Could you check a few things on this model? Use its own coordinates, in mm. A direction names the side the tool comes from. Give positions to 0.01 mm unless a question says otherwise; leave off trailing zeros. Loops run counter-clockwise (first coordinate to the right, second up) from the corner with the lowest first, then second, coordinate; pieces in that order, holes last. Notation, with made-up numbers: (37, 27) - (73, 27) arc R15 ccw to (73, 52) - close; hole circle Ø9 at (52, 12.25). An arc over 180 degrees is marked (long way). Write each question's results on one line, items separated by ' | '. Start each with the question number.
(1) For pin 1 (0.8 mm diameter, centred on x = 3, z = 30.5, fed in from -Y), with a flat end and sliding along its axis, tell me the tip position at first contact or that it passes through.
(2) Suppose I cut it at D-D (y = 6). Count the separate pieces of the cut face and the enclosed holes in it, and give its area (3 significant figures).
(3) On a 3-axis mill with a long thin cutter (end or side, diameter ignored), from which of +Z, -Z, +X, -X, +Y, -Y can I reach the whole of each face in a straight line? I mean faces 3 (the face through (5.5, 14, 29)), 4 (the face through (3, 18, 2)), 5 (the face through (11.5, 7, 30)), 6 (the face through (3, 4.2, 30)), 7 (the face through (3, 10, 4.5)). Say none if no direction works.
(4) Suppose I cut it at B-B (x = 3). Please give me the cut outline in (y, z), and give its area (3 significant figures).
(5) Suppose I cut it at C-C (z = 13.5). Please give me the cut outline in (x, y).
(6) Suppose I cut it at A-A (y = 14.5). Please give me the cut outline in (x, z), and give its area (3 significant figures).
(7) I need wall thicknesses on line 1 (Y direction, x = 1.05, z = 2.25); line 2 (Y direction, x = 8.5, z = 2.25); line 3 (Z direction, x = 4, y = 17.5). Which ranges of each line are inside material? Lowest first, please.
(8) If we mould it in two halves opening along Z, with no side actions, what happens to faces 1 (the face through (12, 18, 2)), 2 (the face through (3, 4.2, 2))? For each: released by +Z, released by -Z, zero draft, split by the parting line, or undercut.
from build123d import *

# Parameters (mm, degrees)
SKETCH_1_W          = 15
SKETCH_1_H          = 32.4
SKETCH_1_R          = 0.8
EXTRUDE_1_DEPTH     = 2.2
SKETCH_2_W          = 15
SKETCH_2_H          = 32.4
SKETCH_2_W_2        = 12.4
SKETCH_2_H_2        = 23.4
EXTRUDE_2_DEPTH     = 15.8
EXTRUDE_START       = 15.8
SKETCH_2_3_W        = 1.3
SKETCH_2_3_H        = 4.5
SKETCH_2_3_H_2      = 23.4
EXTRUDE_3_DEPTH     = 2.5
SKETCH_3_W          = 8
SKETCH_3_H          = 3
SKETCH_3_W_2        = 4
SKETCH_3_H_2        = 1.5
CUT_EXTRUDE_1_DEPTH = 42.170499147
SKETCH_4_R          = 0.5
CUT_EXTRUDE_2_DEPTH = 42.170499147
SKETCH_5_W          = 32.4
SKETCH_5_H          = 2.2
CUT_EXTRUDE_3_DEPTH = 42.170499147
SKETCH_6_R          = 0.5
CUT_EXTRUDE_4_DEPTH = 2
SKETCH_7_W          = 4
SKETCH_7_H          = 1.5
CUT_EXTRUDE_5_DEPTH = 39.461019227


with BuildPart() as part:
    # 草图1 → 凸台-拉伸1 (new body)
    with BuildSketch(Plane(origin=(0, 0, 0), x_dir=(1, 0, 0), z_dir=(0, 1, 0))):
        with Locations((7.5, -16.2)):
            Rectangle(SKETCH_1_W, SKETCH_1_H)
        with Locations(Location((3, -3, 0), (0, 0, 270))):
            Circle(SKETCH_1_R, mode=Mode.SUBTRACT)
        with Locations(Location((12, -3, 0), (0, 0, 270))):
            Circle(SKETCH_1_R, mode=Mode.SUBTRACT)
        with Locations(Location((3, -29.4, 0), (0, 0, 270))):
            Circle(SKETCH_1_R, mode=Mode.SUBTRACT)
        with Locations(Location((12, -29.4, 0), (0, 0, 270))):
            Circle(SKETCH_1_R, mode=Mode.SUBTRACT)
    extrude(amount=EXTRUDE_1_DEPTH)

    # 草图2 → 凸台-拉伸2 (add)
    with BuildSketch(Plane(origin=(0, 2.2, 0), x_dir=(1, 0, 0), z_dir=(0, 1, 0))):
        with Locations((7.5, -16.2)):
            Rectangle(SKETCH_2_W, SKETCH_2_H)
        with Locations((7.5, -16.2)):
            Rectangle(SKETCH_2_W_2, SKETCH_2_H_2, mode=Mode.SUBTRACT)
    extrude(amount=EXTRUDE_2_DEPTH)

    # 草图2<3> → 凸台-拉伸3 (add)
    with BuildSketch(Plane(origin=(0, 2.2, 0), x_dir=(1, 0, 0), z_dir=(0, 1, 0)).offset(EXTRUDE_START)):
        with Locations((0.65, -2.25)):
            Rectangle(SKETCH_2_3_W, SKETCH_2_3_H)
        with Locations((0.65, -16.2)):
            Rectangle(SKETCH_2_3_W, SKETCH_2_3_H_2)
        with Locations((0.65, -30.15)):
            Rectangle(SKETCH_2_3_W, SKETCH_2_3_H)
        with Locations((14.35, -30.15)):
            Rectangle(SKETCH_2_3_W, SKETCH_2_3_H)
        with Locations((14.35, -16.2)):
            Rectangle(SKETCH_2_3_W, SKETCH_2_3_H_2)
        with Locations((14.35, -2.25)):
            Rectangle(SKETCH_2_3_W, SKETCH_2_3_H)
    extrude(amount=EXTRUDE_3_DEPTH)

    # 草图3 → 切除-拉伸1 (cut, through all)
    with BuildSketch(Plane(origin=(0, 0, 0), x_dir=(-1, 0, 0), z_dir=(0, 0, -1))):
        with Locations((-7.5, 6.7)):
            Rectangle(SKETCH_3_W, SKETCH_3_H)
        with Locations((-7.5, 17.25)):
            Rectangle(SKETCH_3_W_2, SKETCH_3_H_2)
    extrude(amount=-CUT_EXTRUDE_1_DEPTH, mode=Mode.SUBTRACT)

    # 草图4 → 切除-拉伸2 (cut, through all)
    with BuildSketch(Plane(origin=(15, 0, 0), x_dir=(0, 0, -1), z_dir=(1, 0, 0))):
        with Locations((-30.15, 6)):
            Circle(SKETCH_4_R)
        with Locations((-2.25, 6)):
            Circle(SKETCH_4_R)
        with Locations((-30.15, 14.5)):
            Circle(SKETCH_4_R)
        with Locations((-2.25, 14.5)):
            Circle(SKETCH_4_R)
    extrude(amount=-CUT_EXTRUDE_2_DEPTH, mode=Mode.SUBTRACT)

    # 草图5 → 切除-拉伸3 (cut, through all)
    with BuildSketch(Plane.ZY):
        with Locations((16.2, 1.1)):
            Rectangle(SKETCH_5_W, SKETCH_5_H)
    extrude(amount=-CUT_EXTRUDE_3_DEPTH, mode=Mode.SUBTRACT)

    # 草图6 → 切除-拉伸4 (cut)
    with BuildSketch(Plane.XZ.offset(-2.2)):
        with Locations(Location((12, 30.15, 0), (0, 0, 270))):
            Circle(SKETCH_6_R)
        with Locations(Location((3, 30.15, 0), (0, 0, 270))):
            Circle(SKETCH_6_R)
        with Locations(Location((12, 2.25, 0), (0, 0, 270))):
            Circle(SKETCH_6_R)
        with Locations(Location((3, 2.25, 0), (0, 0, 270))):
            Circle(SKETCH_6_R)
    extrude(amount=-CUT_EXTRUDE_4_DEPTH, mode=Mode.SUBTRACT)

    # 草图7 → 切除-拉伸5 (cut, through all)
    with BuildSketch(Plane(origin=(0, 16.5, 0), x_dir=(1, 0, 0), z_dir=(0, 1, 0))):
        with Locations((7.5, -28.65)):
            Rectangle(SKETCH_7_W, SKETCH_7_H)
        with Locations((7.5, -3.75)):
            Rectangle(SKETCH_7_W, SKETCH_7_H)
    extrude(amount=-CUT_EXTRUDE_5_DEPTH, mode=Mode.SUBTRACT)


solid = part.part
Output values:
1) pin 1: y = 2.2
2) separate pieces: 6 | enclosed holes: 0 | area: 110 mm2
3) face 3: +Y | face 4: +Z, -Z, +Y | face 5: +Z, -Z | face 6: -Y | face 7: +Y, -Y
4) outline: (2.2, 0) - (18, 0) - (18, 4.5) - (2.2, 4.5) - (2.2, 2.75) - (4.2, 2.75) - (4.2, 1.75) - (2.2, 1.75) - close; (2.2, 27.9) - (18, 27.9) - (18, 32.4) - (2.2, 32.4) - (2.2, 30.65) - (4.2, 30.65) - (4.2, 29.65) - (2.2, 29.65) - close; hole circle Ø1 at (6, 2.25); hole circle Ø1 at (6, 30.15); hole circle Ø1 at (14.5, 2.25); hole circle Ø1 at (14.5, 30.15) | area: 135 mm2
5) outline: (0, 2.2) - (1.3, 2.2) - (1.3, 20.5) - (0, 20.5) - close; (13.7, 2.2) - (15, 2.2) - (15, 20.5) - (13.7, 20.5) - close
6) outline: (0, 0) - (15, 0) - (15, 1.75) - (0, 1.75) - close; (0, 2.75) - (15, 2.75) - (15, 29.65) - (0, 29.65) - close; (0, 30.65) - (15, 30.65) - (15, 32.4) - (0, 32.4) - close; hole (1.3, 4.5) - (5.5, 4.5) - (5.5, 3) - (9.5, 3) - (9.5, 4.5) - (13.7, 4.5) - (13.7, 27.9) - (9.5, 27.9) - (9.5, 29.4) - (5.5, 29.4) - (5.5, 27.9) - (1.3, 27.9) - close | area: 154 mm2
7) line 1: 2.2 to 5.5, 6.5 to 14, 15 to 20.5 | line 2: 2.2 to 5.2, 8.2 to 14, 15 to 16.5 | line 3: 0 to 4.5, 27.9 to 32.4
8) face 1: zero draft | face 2: undercut
